Verification items for the finished model (mm, model axes). Face numbers are marked on the shaded views. A direction names the side the tool comes from. Give positions to 0.01 mm unless a question says otherwise; leave off trailing zeros. Loops run counter-clockwise (first coordinate to the right, second up) from the corner with the lowest first, then second, coordinate; pieces in that order, holes last. Notation, with made-up numbers: (43, -32.5) -> (54, -32.5) arc R19 cw to (54, -11.5) -> close; hole circle Ø8 at (45, -13). An arc over 180 degrees is marked (long way). Use one line per item in the form item = value. Start each with the question number.
from build123d import *

# Parameters (mm, degrees)
F1_DEPTH    = 11
F3_DEPTH    = 11
F5_W        = 8
F5_H        = 38
F6_DEPTH    = 38
F7_T4_DEPTH = 203.4479070854


# Not quite as in the source:
# - a fillet or chamfer that OpenCascade refuses, or shapes differently, is made with other operations: its cross-section is extruded or revolved along the edge and cut away or added


with BuildPart() as f1:
    # F0 (on Front) → F1 (new body)
    with BuildSketch(Plane.XZ):
        with BuildLine():
            Line((0, 38), (0, 0))
            Line((0, 0), (38, 0))
            Line((38, 0), (38, 38))
            ThreePointArc((38, 38), (19, 57), (0, 38))
        make_face()
    extrude(amount=F1_DEPTH)

    # F2 (on Top) → F3 (join)
    with BuildSketch(Plane.XY):
        with BuildLine():
            Line((38, 0), (0, 0))
            Line((0, 0), (0, -38))
            ThreePointArc((0, -38), (19, -57), (38, -38))
            Line((38, -38), (38, 0))
        make_face()
    extrude(amount=F3_DEPTH)

    # F5 (on offset) → F6 (join)
    with BuildSketch(Plane.XZ.offset(11)):
        with Locations((19, 29.9000790417)):
            Rectangle(F5_W, F5_H)
    extrude(amount=F6_DEPTH)

    # F7: chamfer of 38 on 1 edges, made by hand


with BuildPart() as f7_tool2:
    # F7_s3 → F7_t4 (new body)
    with BuildSketch(Plane.YZ.offset(120.7239535427)):
        Polygon((-11, 48.9000790417), (-49, 10.9000790417), (-49, 48.9000790417), align=None)
    extrude(amount=-F7_T4_DEPTH)

    split(bisect_by=Plane.XZ.offset(11), keep=Keep.TOP)

    split(bisect_by=Plane.XY.offset(11), keep=Keep.TOP)


with BuildPart() as f1_1:
    add(f1.part)

    # F7_t1: cut F7_tool2
    add(f7_tool2.part, mode=Mode.SUBTRACT)


solid = f1_1.part
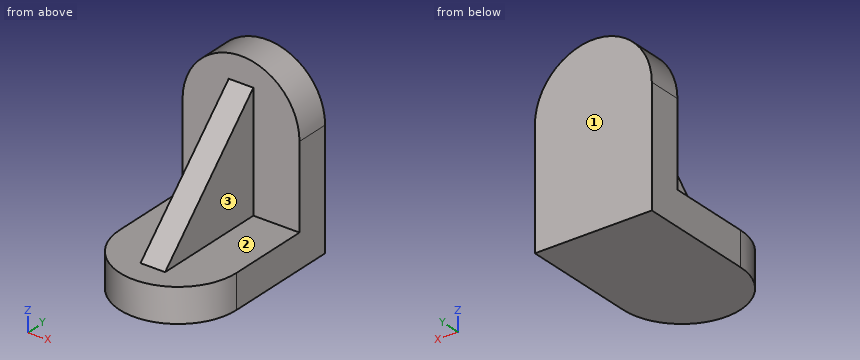
Item 1: Sectioned sample at D-D, the plane x = 10. Enter the section's corners in (y, z), and give its area (3 significant figures).
Item 2: Material ranges on line 1 (Z direction, x = 13, y = -44.5); line 2 (X direction, y = -19, z = 21.5); line 3 (Y direction, x = 30, z = 19), recorded low to high.
Item 3: Tool access check on the marked faces 1, 2 and 3. Record the directions out of +Z, -Z, +X, -X, +Y, -Y that give a thin tool (end or side, any length) a straight path to the whole face; none if there is none.
Item 4: Sectioned sample at C-C, the plane y = -18. Enter the section's corners in (x, z).
Item 5: Sectioned sample at A-A, the plane x = 19. Enter the section's corners in (y, z), and give its area (3 significant figures).
Item 6: Gauge pin test, flat ends, axial feed: pin 1 Ø10 at (x, z) = (31, 48.5) entering from -Y; pin 2 Ø5 at (x, y) = (14.5, -23.5) entering from -Z; pin 3 Ø11.5 at (y, z) = (-26.5, 26.5) entering from -X; pin 4 Ø6 at (x, y) = (7, -13) entering from +Z. Record the tip position at first contact, or that the pin passes through.
Item 7: Sectioned sample at B-B, the plane z = 14. Enter the section's corners in (x, y), and give its area (3 significant figures).
Outcome:
q1.outline = (-54.73, 0) -> (0, 0) -> (0, 54.73) -> (-11, 54.73) -> (-11, 11) -> (-54.73, 11) -> close
q1.area = 1,080 mm^2
q2.line_1 = 0 to 11
q2.line_2 = 15 to 23
q2.line_3 = -11 to 0
q3.face_1 = +Z, -Z, +X, -X, +Y
q3.face_2 = +Z, -Y
q3.face_3 = +Z, +X, -Y
q4.outline = (0, 0) -> (38, 0) -> (38, 11) -> (23, 11) -> (23, 41.9) -> (15, 41.9) -> (15, 11) -> (0, 11) -> close
q5.outline = (-57, 0) -> (0, 0) -> (0, 57) -> (-11, 57) -> (-11, 48.9) -> (-48.9, 11) -> (-57, 11) -> close
q5.area = 1,850 mm^2
q6.pin_1 = -11
q6.pin_2 = 0
q6.pin_3 = 15
q6.pin_4 = 54.3
q7.outline = (0, -11) -> (15, -11) -> (15, -45.9) -> (23, -45.9) -> (23, -11) -> (38, -11) -> (38, 0) -> (0, 0) -> close
q7.area = 697 mm^2
